Geometry: final body of the model. Coordinates: model frame, mm. Face numbers are marked on the shaded views. Round coordinates to 2 decimals unless told otherwise and drop trailing zeros. Loops run counter-clockwise (first coordinate to the right, second up) from the corner with the lowest first, then second, coordinate; pieces in that order, holes last. Notation, with made-up numbers: M 13,-13.75 L 54,-13.75 A16 ccw 54,-6.75 Z; hole C 66,-4.75 d8. An arc over 180 degrees is marked long. Return JSON: item names as keys, results as strings.
from build123d import *

# Parameters (mm, degrees)
SKETCH2_R           = 100
BOSS_EXTRUDE1_DEPTH = 2.5
CUT_EXTRUDE1_DEPTH  = 2.5
CUT_EXTRUDE2_DEPTH  = 10
SKETCH6_R           = 7.5
SKETCH6_R_2         = 7
CUT_EXTRUDE3_DEPTH  = 10


with BuildPart() as part:
    # Sketch2 → Boss-Extrude1 (new, symmetric)
    with BuildSketch(Plane(origin=(0, 0, 0), x_dir=(1, 0, 0), z_dir=(0, 1, 0))):
        with Locations(Location((0, 0, 0), (0, 0, 270))):
            Circle(SKETCH2_R)
    extrude(amount=BOSS_EXTRUDE1_DEPTH, both=True)

    # Sketch3 → Cut-Extrude1 (cut)
    with BuildSketch(Plane.XZ.offset(2.5)):
        Polygon((-65, 0), (-65, -50), (-55, -50), (-55, 50), (-65, 50), align=None)
        Polygon((55, 50), (65, 50), (65, 0), (65, -50), (55, -50), align=None)
    extrude(amount=-CUT_EXTRUDE1_DEPTH, mode=Mode.SUBTRACT)

    # Sketch5 → Cut-Extrude2 (cut)
    with BuildSketch(Plane.XZ.offset(2.5)):
        Polygon((0, 30.36), (10, 30.36), (10, -10.14), (-10, -10.14), (-10, 30.36), align=None)
    extrude(amount=-CUT_EXTRUDE2_DEPTH, mode=Mode.SUBTRACT)

    # Sketch6 → Cut-Extrude3 (cut)
    with BuildSketch(Plane.XZ.offset(2.5)):
        with Locations(Location((-45, 0, 0), (0, 0, 270))):
            Circle(SKETCH6_R)
        with Locations(Location((0, -45, 0), (0, 0, 270))):
            Circle(SKETCH6_R)
        with Locations(Location((45, 0, 0), (0, 0, 270))):
            Circle(SKETCH6_R)
        with Locations(Location((0, 55, 0), (0, 0, 270))):
            Circle(SKETCH6_R_2)
    extrude(amount=-CUT_EXTRUDE3_DEPTH, mode=Mode.SUBTRACT)


solid = part.part
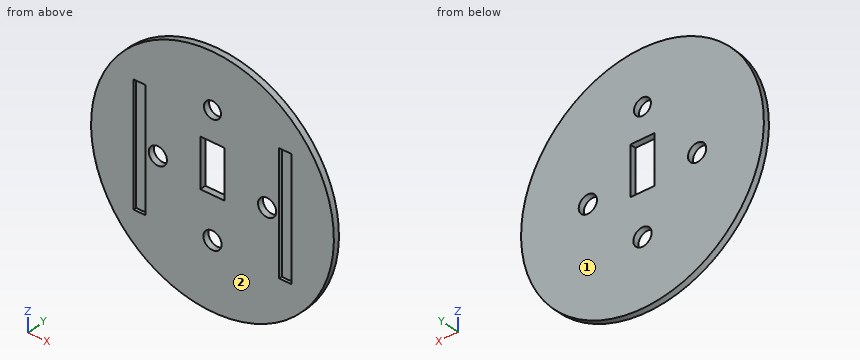
Q1. Pull-direction query (Y, two-part tool) for the marked faces 1 and 2; classes: pulls with the +Y half, pulls with the -Y half, needs draft (parallel to the pull), parting line crosses it, or undercut.
Determined:
{"face 1": "pulls with the +Y half", "face 2": "pulls with the -Y half"}
Q2. Pin query (flat end, axial travel): pin 1 (3 mm diameter, centred on x = -59.5, z = 11, fed in from -Y); pin 2 (1 mm diameter, centred on x = -58.5, y = 1, fed in from +Z); pin 3 (3 mm diameter, centred on y = -2, z = -15, fed in from +X); pin 4 (24 mm diameter, centred on x = -45, z = 0, fed in from -Y). Return the tip coordinate at first contact, or that it passes through.
Determined:
{"pin 1": "stops at y = 0", "pin 2": "stops at z = 81.46", "pin 3": "stops at x = 99.08", "pin 4": "stops at y = -2.5"}
Q3. Section query A-A (x = 0). Output: boundary loops of the cut face in (y, z), plus the area to 4 significant figures.
Determined:
{"outline": "M -2.5,-100 L 2.5,-100 L 2.5,-52.5 L -2.5,-52.5 Z; M -2.5,-37.5 L 2.5,-37.5 L 2.5,-10.14 L -2.5,-10.14 Z; M -2.5,30.36 L 2.5,30.36 L 2.5,48 L -2.5,48 Z; M -2.5,62 L 2.5,62 L 2.5,100 L -2.5,100 Z", "area": "652.5 mm^2"}
Q4. Section query B-B (z = 0). Output: boundary loops of the cut face in (x, y).
Determined:
{"outline": "M -100,-2.5 L -65,-2.5 L -65,0 L -55,0 L -55,-2.5 L -52.5,-2.5 L -52.5,2.5 L -100,2.5 Z; M -37.5,-2.5 L -10,-2.5 L -10,2.5 L -37.5,2.5 Z; M 10,-2.5 L 37.5,-2.5 L 37.5,2.5 L 10,2.5 Z; M 52.5,-2.5 L 55,-2.5 L 55,0 L 65,0 L 65,-2.5 L 100,-2.5 L 100,2.5 L 52.5,2.5 Z"}
Q5. Material intervals for L1, parallel to X at y = -0.6, z = 0; L2, parallel to X at y = 0.7, z = 0; L3, parallel to X at y = 1.2, z = -4.5, sorted ascending.
Determined:
{"L1": "x = -100 to -65, -55 to -52.5, -37.5 to -10, 10 to 37.5, 52.5 to 55, 65 to 100", "L2": "x = -100 to -52.5, -37.5 to -10, 10 to 37.5, 52.5 to 100", "L3": "x = -99.9 to -51, -39 to -10, 10 to 39, 51 to 99.9"}
Q6. Section query D-D (y = -1). Output: boundary loops of the cut face in (x, z), plus the area to 3 significant figures.
Determined:
{"outline": "C 0,0 d200; hole M -65,-50 L -55,-50 L -55,50 L -65,50 Z; hole C -45,0 d15; hole M -10,-10.14 L 10,-10.14 L 10,30.36 L -10,30.36 Z; hole C 0,-45 d15; hole C 0,55 d14; hole C 45,0 d15; hole M 55,-50 L 65,-50 L 65,50 L 55,50 Z", "area": "27,900 mm^2"}
Q7. Section query C-C (z = -45). Output: boundary loops of the cut face in (x, y).
Determined:
{"outline": "M -89.3,-2.5 L -65,-2.5 L -65,0 L -55,0 L -55,-2.5 L -7.5,-2.5 L -7.5,2.5 L -89.3,2.5 Z; M 7.5,-2.5 L 55,-2.5 L 55,0 L 65,0 L 65,-2.5 L 89.3,-2.5 L 89.3,2.5 L 7.5,2.5 Z"}
